Can you work these out from the model? Positions are in its coordinate system, mm. A direction names the side the tool comes from. Give positions to 0.01 mm unless a question says otherwise; leave off trailing zeros. Loops run counter-clockwise (first coordinate to the right, second up) from the corner with the lowest first, then second, coordinate; pieces in that order, holes last. Notation, with made-up numbers: (65.5, 70) - (71.5, 70) arc R32 cw to (71.5, 105) - close; hole circle Ø10 at (79, -25.75). An arc over 180 degrees is marked (long way). Answer as a JSON object with one key per item and string values.
```python
from build123d import *

# Parameters (mm, degrees)
F0_W      = 76.2
F0_H      = 127
F1_DEPTH  = 6.35
F2_W      = 10.16
F2_H      = 6.35
F3_DEPTH  = 25.4
F5_DEPTH  = 76.2
F7_DEPTH  = 38.1
F8_W      = 55.88
F8_H      = 9.9150016904
F9_DEPTH  = 6.35
F11_R     = 2.54
F12_DEPTH = 27.94


with BuildPart() as f1:
    # F0 (on Top) → F1 (new body)
    with BuildSketch(Plane.XY):
        Rectangle(F0_W, F0_H)
    extrude(amount=F1_DEPTH)

    # F2 (on face) → F3 (cut)
    with BuildSketch(Plane.XY.offset(6.35)):
        with Locations((-33.02, -60.325)):
            Rectangle(F2_W, F2_H)
        with Locations((33.02, -60.325)):
            Rectangle(F2_W, F2_H)
    extrude(amount=-F3_DEPTH, mode=Mode.SUBTRACT)

    # F4 (on face) → F5 (cut)
    with BuildSketch(Plane(origin=(-27.94, 0, 0), x_dir=(0, -1, 0), z_dir=(-1, 0, 0))):
        with BuildLine():
            ThreePointArc((60.325, 6.35), (62.5700640303, 5.4200640303), (63.5, 3.175))
            Line((63.5, 3.175), (63.5, 6.35))
            Line((63.5, 6.35), (60.325, 6.35))
        make_face()
        with BuildLine():
            Line((63.5, 0), (63.5, 3.175))
            ThreePointArc((63.5, 3.175), (62.5700640303, 0.9299359697), (60.325, 0))
            Line((60.325, 0), (63.5, 0))
        make_face()
    extrude(amount=-F5_DEPTH, mode=Mode.SUBTRACT)

    # F6 (on Right) → F7 (cut, symmetric)
    with BuildSketch(Plane.YZ):
        with BuildLine():
            Line((-57.15, 6.35), (-57.15, 0))
            ThreePointArc((-57.15, 0), (-53.975, 3.175), (-57.15, 6.35))
        make_face()
    extrude(amount=F7_DEPTH, both=True, mode=Mode.SUBTRACT)

    # F8 (on Top) → F9 (join)
    with BuildSketch(Plane.XY):
        with Locations((0, -52.1924991548)):
            Rectangle(F8_W, F8_H)
    extrude(amount=F9_DEPTH)

    # F11 (on Right) → F12 (cut, symmetric)
    with BuildSketch(Plane.YZ):
        with Locations((-57.15, 3.175)):
            Circle(F11_R)
    extrude(amount=F12_DEPTH, both=True, mode=Mode.SUBTRACT)


solid = f1.part
```
1) I need wall thicknesses on L1, parallel to Z at x = 3.5, y = -57.15 (3 decimals); L2, parallel to Y at x = 3, z = 4; L3, parallel to Y at x = 19, z = 1.5. Which ranges of each line are inside material? Lowest first, please.
Check sheet entries:
{"L1": "0 to 0.635, 5.715 to 6.35", "L2": "-63.39 to -59.55, -54.75 to 63.5", "L3": "-63.02 to -59.06, -55.24 to 63.5"}
2) If we mould it in two halves opening along Z, with no side actions, what happens to faces 1 (the flat face through (-1, 63.5, 3)), 2 (the flat face through (-1, 2, 6.35)), 3 (the cylindrical face through (33.091, -53.976, 3.105)), 4 (the flat face through (-1, 2, 0))? For each: released by +Z, released by -Z, zero draft, split by the parting line, or undercut.
Check sheet entries:
{"face 1": "zero draft", "face 2": "released by +Z", "face 3": "undercut", "face 4": "released by -Z"}
3) Imagine slicing it at A-A on x = -15.5. Write out the boundary of the cut face in (y, z) (3 decimals), and give its area (3 significant figures).
Check sheet entries:
{"outline": "(-60.325, 0) - (63.5, 0) - (63.5, 6.35) - (-60.325, 6.35) arc R3.175 ccw to start; hole circle Ø5.08 at (-57.15, 3.175)", "area": "782 mm2"}
4) I'm going to push flat-ended pins straight in: P1, Ø3, axis at y = -57.15, z = 3.175, coming from the -X side; P2, Ø1.9, axis at y = -58, z = 1.5, coming from the -X side. Where does each tip first touch, or does it pass through?
Check sheet entries:
{"P1": "through", "P2": "x = -27.94"}
5) Which directions (+Z, -Z, +X, -X, +Y, -Y) give clear straight access to the entire face, cutting with the end or side of a thin tool? Please do faces 5 (the flat face through (27.94, -60, 3)), 6 (the cylindrical face through (0.39, -54.73, 3.94)), 7 (the flat face through (-27.94, -60, 3)).
Check sheet entries:
{"face 5": "+X, -Y", "face 6": "+X, -X", "face 7": "-X, -Y"}
6) Imagine slicing it at B-B on z = 4.5. Write out the boundary of the cut face in (x, y), and give its area (3 significant figures).
Check sheet entries:
{"outline": "(-38.1, -54.26) - (-27.94, -54.26) - (-27.94, -54.98) - (27.94, -54.98) - (27.94, -54.26) - (38.1, -54.26) - (38.1, 63.5) - (-38.1, 63.5) - close; (-27.94, -63.21) - (27.94, -63.21) - (27.94, -59.32) - (-27.94, -59.32) - close", "area": "9,230 mm2"}
